Here's how the part is built. I have some questions about the finished solid (model axes, mm). A direction names the side the tool comes from. Coordinates: 2 decimals unless noted, no trailing zeros. Write each loop counter-clockwise with the first axis right and the second up, starting at its lowest first coordinate (ties: lowest second). Pieces come first, ordered by that corner, then holes. Notation, with made-up numbers: (-30, 65.25) -> (-3, 65.25) arc R18 cw to (-3, 78.25) -> close; hole circle Ø9 at (76.5, 12.25). An arc over 180 degrees is marked (long way). Answer in a Markdown table with one row per item. Add a question column.
from build123d import *

# Parameters (mm, degrees)
SKETCH2_W                  = 30
SKETCH2_H                  = 12.7
CUT_EXTRUDE1_DEPTH         = 1.5
F_8_32_TAPPED_HOLE1_D      = 3.4544
F_8_32_TAPPED_HOLE1_DEPTH  = 10.71
F_8_32_TAPPED_HOLE1_TIP    = 1.037806461
SKETCH7_OUTSIDE_W          = 29.718
SKETCH7_OUTSIDE_H          = 31.218
SKETCH7_OUTSIDE_R          = 6.6
CUT_EXTRUDE2_DEPTH         = 2
F_3_8_0_3750_DOWEL_HOLE2_D = 9.525
CUT_EXTRUDE4_START         = 9
SKETCH11_W                 = 18
SKETCH11_H                 = 20
CUT_EXTRUDE4_DEPTH         = 1
F_1_4_0_2500_DOWEL_HOLE1_D = 6.35
CHAMFER1_SIZE              = 0.5


with BuildPart() as part:
    # Sketch1 → Revolve1 (revolve)
    with BuildSketch(Plane(origin=(0, 0, 0), x_dir=(1, 0, 0), z_dir=(0, 1, 0)), mode=Mode.PRIVATE) as revolve1_sk:
        Polygon((-21.5, 0), (29, 0), (29, 4), (13.5, 4), (13.5, 9), (-15, 9), (-15, 4), (-21.5, 4), align=None)
    revolve(revolve1_sk.sketch.rotate(Axis((-21.5, 0, 0), (1, 0, 0)), 180), axis=Axis((-21.5, 0, 0), (1, 0, 0)))

    # Sketch2 → Cut-Extrude1 (cut)
    with BuildSketch(Plane.XY.offset(9)):
        Rectangle(SKETCH2_W, SKETCH2_H)
    extrude(amount=-CUT_EXTRUDE1_DEPTH, mode=Mode.SUBTRACT)

    # #8-32 Tapped Hole1
    with Locations(Plane.ZY.offset(21.5)):
        with Locations((0, 0)):
            Hole(F_8_32_TAPPED_HOLE1_D / 2, depth=F_8_32_TAPPED_HOLE1_DEPTH)
            with Locations((0, 0, -(F_8_32_TAPPED_HOLE1_DEPTH + F_8_32_TAPPED_HOLE1_TIP / 2))):  # 118° drill point
                Cone(0, F_8_32_TAPPED_HOLE1_D / 2, F_8_32_TAPPED_HOLE1_TIP, mode=Mode.SUBTRACT)

    # Sketch7 outside → Cut-Extrude2 (cut)
    with BuildSketch(Plane.ZY.offset(15)):
        with Locations((-0.75, 0)):
            Rectangle(SKETCH7_OUTSIDE_W, SKETCH7_OUTSIDE_H)
        Circle(SKETCH7_OUTSIDE_R, mode=Mode.SUBTRACT)
    extrude(amount=-CUT_EXTRUDE2_DEPTH, mode=Mode.SUBTRACT)

    # 3/8 (0.3750) Dowel Hole2 (through all)
    with Locations(Plane.XY.offset(7.5)):
        with Locations((0, 0)):
            Hole(F_3_8_0_3750_DOWEL_HOLE2_D / 2)

    # Sketch11 → Cut-Extrude4 (cut)
    with BuildSketch(Plane(origin=(0, 0, 0), x_dir=(1, 0, 0), z_dir=(0, 1, 0)).offset(CUT_EXTRUDE4_START)):
        Rectangle(SKETCH11_W, SKETCH11_H)
    cut_extrude4 = extrude(amount=-CUT_EXTRUDE4_DEPTH, mode=Mode.SUBTRACT)

    # 1/4 (0.2500) Dowel Hole1 (through all)
    with Locations(Plane(origin=(0, 8, 0), x_dir=(1, 0, 0), z_dir=(0, 1, 0))):
        with Locations((0, 0)):
            Hole(F_1_4_0_2500_DOWEL_HOLE1_D / 2)

    # Mirror1: Cut-Extrude4 across plane
    add(cut_extrude4.mirror(Plane.ZX), mode=Mode.SUBTRACT)

    # Chamfer1
    chamfer1_edges = [part.edges().sort_by_distance(p)[0] for p in [
        (3.175, 8, 0),
    ]]
    chamfer(chamfer1_edges, length=CHAMFER1_SIZE)


solid = part.part
Q1. If we mould it in two halves opening along X, with no side actions, what happens to faces 4 (the flat face through (29, 0, 0)), 5 (the flat face through (-9, 8.4, 0.1)), 6 (the cylindrical face through (21.142, 3.905, -0.867))? For each: pulls with the +X half, pulls with the -X half, needs draft (parallel to the pull), parting line crosses it, or undercut.
Q2. Imagine slicing it at C-C on x = 7. Please give me the cut outline in (y, z).
Q3. Imagine slicing it at B-B on y = -5.75. Please give me the cut outline in (x, z) (3 decimals), plus the area to 3 significant figures.
Q4. Imagine slicing it at A-A on z = -7.5. Please give me the cut outline in (x, y) (1 decimal).
Q5. For faces 1 (the flat face through (9, -8.4, 0.1)), 2 (the flat face through (-15, 3, 3)), 3 (the flat face through (-4, 8, 0)), which set-ups out of +Z, -Z, +X, -X, +Y, -Y let a thin tool reach every point of the face, with its end or its side?
Q6. I'm going to push flat-ended pins straight in: P1, Ø6.5, axis at x = 0, z = 2, coming from the -Y side; P2, Ø0.5, axis at y = -8.5, z = -1, coming from the +X side; P3, Ø9, axis at x = 1, z = -1, coming from the +Y side. Where does each tip first touch, or does it pass through?
Q7. I need wall thicknesses on line 1 (X direction, y = 5.05, z = 0) (3 decimals); line 2 (Z direction, x = -1, y = 5.5); line 3 (X direction, y = 6.75, z = -2.5). Which ranges of each line are inside material? Lowest first, please. Write a range as [from, to].
Q8. Imagine slicing it at D-D on x = 0. State how many separate pieces and enclosed holes the cut face has, plus the area to 3 significant figures.
Result sheet:
| question | item | result |
|---|---|---|
| 1 | face 4 | pulls with the +X half |
| 1 | face 5 | undercut |
| 1 | face 6 | needs draft |
| 2 | outline | (-8, -4.12) arc R9 ccw to (8, -4.12) -> (8, 4.12) arc R9 ccw to (4.97, 7.5) -> (-4.97, 7.5) arc R9 ccw to (-8, 4.12) -> close |
| 3 | outline | (-15, -3.24) -> (-13, -3.24) -> (-13, -6.924) -> (13.5, -6.924) -> (13.5, 6.924) -> (-13, 6.924) -> (-13, 3.24) -> (-15, 3.24) -> close; hole circle Ø6.35 at (0, 0) |
| 3 | area | 348 mm^2 |
| 4 | outline | (-13, -5) -> (13.5, -5) -> (13.5, 5) -> (-13, 5) -> close; hole circle Ø9.5 at (0, 0) |
| 5 | face 1 | +Z, -Z, -Y |
| 5 | face 2 | -X |
| 5 | face 3 | +Z, -Z, +Y |
| 6 | P1 | stops at y = -8 |
| 6 | P2 | stops at x = 13.5 |
| 6 | P3 | stops at y = 8 |
| 7 | line 1 | x = [-15, -3.175], [3.175, 13.5] |
| 7 | line 2 | z = [-7.12, -3.01], [3.01, 7.12] |
| 7 | line 3 | x = [-13, -1.96], [1.96, 13.5] |
| 8 | separate pieces | 4 |
| 8 | enclosed holes | 0 |
| 8 | area | 38.9 mm^2 |
